```python
from build123d import *

# Parameters (mm, degrees)
SKETCH1_R           = 2.5
BOSS_EXTRUDE1_DEPTH = 30
SKETCH2_R           = 4
BOSS_EXTRUDE2_DEPTH = 2.5
CHAMFER1_SIZE       = 1


with BuildPart() as part:
    # Sketch1 → Boss-Extrude1 (new body)
    with BuildSketch(Plane(origin=(0, 0, 0), x_dir=(1, 0, 0), z_dir=(0, 1, 0))):
        Circle(SKETCH1_R)
    extrude(amount=BOSS_EXTRUDE1_DEPTH)

    # Sketch2 → Boss-Extrude2 (add)
    with BuildSketch(Plane(origin=(0, 30, 0), x_dir=(1, 0, 0), z_dir=(0, 1, 0))):
        Circle(SKETCH2_R)
    extrude(amount=BOSS_EXTRUDE2_DEPTH)

    # Chamfer1
    chamfer1_edges = [part.edges().sort_by_distance(p)[0] for p in [
        (-2.5, 30, 0),
    ]]
    chamfer(chamfer1_edges, length=CHAMFER1_SIZE)


solid = part.part
```
CAD build for the part. Positions are in the model's coordinates, mm. A direction names the side the tool comes from. Round coordinates to 2 decimals unless told otherwise and drop trailing zeros. Loops run counter-clockwise (first coordinate to the right, second up) from the corner with the lowest first, then second, coordinate; pieces in that order, holes last. Notation, with made-up numbers: M -23,29.25 L -18,29.25 A26 ccw -18,46.25 Z; hole C -13.5,53.25 d5. An arc over 180 degrees is marked long. Return JSON: item names as keys, results as strings. Group by question number.
(1) Tool access for faces 1 (the flat face through (0, 32.5, 0)), 2 (the cylindrical face through (-0.54, 14.3, 2.44)): list every direction of +Z, -Z, +X, -X, +Y, -Y with a clear straight run to the whole face (end or side of a thin tool).
(2) Drop flat-ended pins along their axis: P1, Ø1, axis at x = -2.5, y = 5, coming from the +Z side; P2, Ø1, axis at y = 4.5, z = 1, coming from the -X side; P3, Ø1.5, axis at x = 2.5, z = 3, coming from the -Y side. Give the stop position or say it passes through.
(3) Saw through at B-B, the plane x = 0. List the corners of the cut face in (y, z), and give its area (3 significant figures).
(4) Wall check: probe 1 along Y at (x, z) = (3.5, -1); probe 2 along X at (y, z) = (31.5, 3.25); probe 3 along Z at (x, y) = (-0.5, 10.5). Give the ranges that are in metal, low to high. Write a range as [from, to].
(5) Saw through at A-A, the plane z = 0. List the corners of the cut face in (x, y), and give its area (3 significant figures).
(6) Saw through at C-C, the plane y = 13.5. List the corners of the cut face in (x, z), and give its area (3 significant figures).
Answer list:
{
 "1": {"face 1": "+Z, -Z, +X, -X, +Y", "face 2": "-Y"},
 "2": {"P1": "z = 1.5", "P2": "x = -2.45", "P3": "y = 29.66"},
 "3": {"outline": "M 0,-2.5 L 29,-2.5 L 30,-3.5 L 30,-4 L 32.5,-4 L 32.5,4 L 30,4 L 30,3.5 L 29,2.5 L 0,2.5 Z", "area": "171 mm2"},
 "4": {"probe 1": "[30, 32.5]", "probe 2": "[-2.33, 2.33]", "probe 3": "[-2.45, 2.45]"},
 "5": {"outline": "M -4,30 L -3.5,30 L -2.5,29 L -2.5,0 L 2.5,0 L 2.5,29 L 3.5,30 L 4,30 L 4,32.5 L -4,32.5 Z", "area": "171 mm2"},
 "6": {"outline": "C 0,0 d5", "area": "19.6 mm2"}
}
